Verification items for the finished model (mm, model axes). Face numbers are marked on the shaded views. A direction names the side the tool comes from. Coordinates: 2 decimals unless noted, no trailing zeros. Order: outer loops, then holes, each group sorted by start corner. A loop starts at its lowest first (then second) coordinate and runs counter-clockwise, first axis right, second up. Notation, with made-up numbers: (28, 28) -> (48, 28) arc R32 ccw to (48, 61) -> close; hole circle Ø1 at (18.25, 77.25). An arc over 180 degrees is marked (long way). Write item = value, one per line. Start each with the question number.
1. Cross-section at C-C on z = -14.5. Record the cut outline in (x, y), plus the area to 3 significant figures.
2. Set-up check for the marked faces 1, 2, 3, 4 and 5: record each of +Z, -Z, +X, -X, +Y, -Y from which the full face is reachable in a straight line by a thin tool's end or side.
3. Thickness scan on line 1 along Z through (x, y) = (-10.5, -35); line 2 along Y through (x, z) = (-43, -63.5); line 3 along X through (y, z) = (45.5, -47). Record the ranges inside material, lowest first. Write a range as from..to.
4. Cross-section at A-A on y = 0. Record the cut outline in (x, z).
5. Cross-section at B-B on x = -48. Record the cut outline in (y, z), plus the area to 3 significant figures.
6. Cross-section at D-D on x = -27. Record the cut outline in (y, z).
7. Release check for a two-part mould opening along Y. For the marked faces 6, 7 and 8 record: +Y half, -Y half, draft (parallel to the pull), parting line (faces both ways), or undercut.
8. Go/stop test with flat-tipped pins: P1, Ø5, axis at x = -48, z = -7, coming from the -Y side; P2, Ø8, axis at x = -28, y = -24.5, coming from the +Z side; P3, Ø2, axis at x = -53, z = -68, coming from the -Y side. Record where each tip stops, or that it passes through.
from build123d import *

# Parameters (mm, degrees)
DODANIE_WYCI_GNI_CIE1_DEPTH       = 25
DODANIE_WYCI_GNI_CIE2_DEPTH       = 5
WYCI_GNI_CIE_CIENKA_CIANKA1_DEPTH = 70
ZAOKR_GLENIE2_R                   = 10


with BuildPart() as part:
    # Szkic1 → Dodanie-wyci_gni_cie1 (new body)
    with BuildSketch(Plane.XY):
        with BuildLine():
            Line((0, -5), (0, -20))
            ThreePointArc((0, -20), (-20, 0), (0, 20))
            Line((0, 20), (0, 5))
            ThreePointArc((0, 5), (-5, 0), (0, -5))
        make_face()
    extrude(amount=DODANIE_WYCI_GNI_CIE1_DEPTH)

    # Szkic2 → Dodanie-wyci_gni_cie2 (add)
    with BuildSketch(Plane.XY):
        with BuildLine():
            Line((0, 20), (0, 72))
            Line((0, 72), (-40, 72))
            Line((-40, 72), (-40, 44.72135955))
            ThreePointArc((-40, 44.72135955), (-56.050341538, -21.409325386), (0, -60))
            Line((0, -60), (0, -20))
            ThreePointArc((0, -20), (-20, 0), (0, 20))
        make_face()
    extrude(amount=DODANIE_WYCI_GNI_CIE2_DEPTH)


with BuildPart() as body_2:
    # Lustro3: mirrored copy
    add(part.part.mirror(Plane(origin=(0, 0, -35), x_dir=(1, 0, 0), z_dir=(0, 0, -1))))


with BuildPart() as part_1:
    add(part.part)

    add(body_2.part)  # Wyci_gni_cie-cienka _cianka1 merges body 2
    # Szkic5 → Wyci_gni_cie-cienka _cianka1 (add)
    with BuildSketch(Plane(origin=(0, 0, 0), x_dir=(-1, 0, 0), z_dir=(0, 0, -1))):
        with BuildLine():
            Line((40, 72), (40, 44.72135955))
            ThreePointArc((40, 44.72135955), (56.050341538, -21.409325386), (0, -60))
            Line((0, -60), (0, -55))
            ThreePointArc((0, -55), (51.76124215, -18.594994247), (35, 42.426406871))
            Line((35, 42.426406871), (35, 72))
            Line((35, 72), (40, 72))
        make_face()
    extrude(amount=WYCI_GNI_CIE_CIENKA_CIANKA1_DEPTH)

    # Zaokr_glenie2
    zaokr_glenie2_edges = [part_1.edges().sort_by_distance(p)[0] for p in [
        (-40, 58.360679775, 5),
        (-35, 57.213203436, -70),
        (-35, 57.213203436, 0),
        (-40, 58.360679775, -75),
    ]]
    fillet(zaokr_glenie2_edges, radius=ZAOKR_GLENIE2_R)


solid = part_1.part
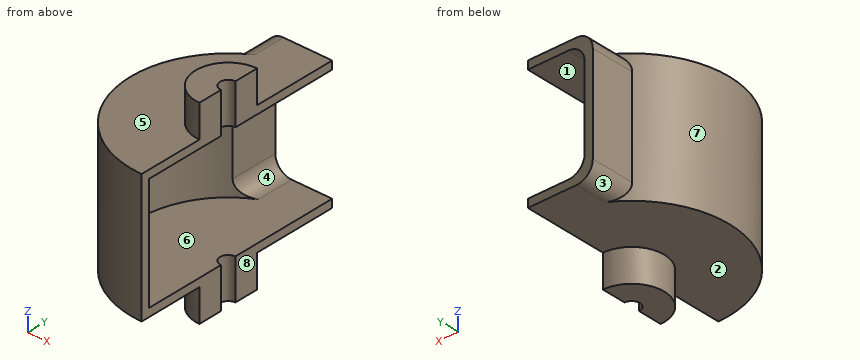
Worked out:
q1.outline = (-40, 44.72) arc R60 ccw to (0, -60) -> (0, -55) arc R55 cw to (-35, 42.43) -> (-35, 72) -> (-40, 72) -> close
q1.area = 841 mm²
q2.face_1 = +X
q2.face_2 = -Z, -X
q2.face_3 = -Z, -X, +Y
q2.face_4 = +X, +Y
q2.face_5 = +Z, -X
q3.line_1 = -75..-70, 0..5
q3.line_2 = -41.84..-34.29, 34.29..41.84
q3.line_3 = -40..-35
q4.outline = (-60, -75) -> (-20, -75) -> (-20, -95) -> (-5, -95) -> (-5, -70) -> (-55, -70) -> (-55, 0) -> (-5, 0) -> (-5, 25) -> (-20, 25) -> (-20, 5) -> (-60, 5) -> close
q5.outline = (-36, -75) -> (36, -75) -> (36, 5) -> (-36, 5) -> close; hole (-26.85, -70) -> (26.85, -70) -> (26.85, 0) -> (-26.85, 0) -> close
q5.area = 2,000 mm²
q6.outline = (-53.58, -75) -> (72, -75) -> (72, -69.8) -> (47.92, -69.8) -> (47.92, -70) -> (-47.92, -70) -> (-47.92, 0) -> (47.92, 0) -> (47.92, -0.2) -> (72, -0.2) -> (72, 5) -> (-53.58, 5) -> close
q7.face_6 = undercut
q7.face_7 = parting line
q7.face_8 = draft
q8.P1 = -39.11
q8.P2 = 5
q8.P3 = -29.93
